Autodesk Inventor part; units mm, degrees
ref_plane "YZ Plane" through (0, 0, 0) normal (1, 0, 0) x (0, 1, 0)
ref_plane "XZ Plane" through (0, 0, 0) normal (0, 1, 0) x (-1, 0, 0)
ref_plane "XY Plane" through (0, 0, 0) normal (0, 0, 1) x (1, 0, 0)
sketch "Sketch1" plane through (0, 0, 0) normal (0, 0, 1) x (1, 0, 0)
  line L0 (0, 0) -> (150, 0)
  line L1 (150, 0) -> (150, -774)
  line L2 (150, -774) -> (0, -774)
  line L3 (0, -774) -> (0, 0)
  dimension "d0" = 150
  dimension "d1" = 774
extrude "Extrusion1" add sketch "Sketch1" along normal blind 4
sketch "Sketch2" plane through (0, 0, 4) normal (0, 0, 1) x (1, 0, 0)
  line L0 (0, 0) -> (0, -774)
  line L1 (0, -150) -> (150, -150)
  line L2 (150, -774) -> (150, 0)
  line L3 (0, -156) -> (150, -156)
  line L4 (150, 0) -> (0, 0)
  line L5 (0, -306) -> (150, -306)
  line L6 (0, -312) -> (150, -312)
  line L7 (0, -462) -> (150, -462)
  line L8 (0, -468) -> (150, -468)
  line L9 (0, -618) -> (150, -618)
  line L10 (0, -624) -> (150, -624)
  line L11 (0, -774) -> (150, -774)
  line L12 (0, -780) -> (150, -780)
  line L13 (75, 0) -> (75, -774)
  line L14 (0, -774) -> (150, -774)
  line L15 (0, 0) -> (0, -774)
  point P0 (75, -306)
  point P1 (75, -618)
  point P2 (75, -156)
  point P3 (75, -150)
  point P4 (75, -312)
  point P5 (75, -306)
  point P6 (75, -468)
  point P7 (75, -462)
  point P8 (75, -624)
  point P9 (75, -618)
  point P10 (75, -780)
  point P11 (75, -774)
  dimension "d4" = 150
  dimension "d5" = 6
  dimension "d6" = 150
  dimension "d8" = 6
  dimension "d9" = 150
  dimension "d10" = 6
  dimension "d11" = 150
  dimension "d12" = 6
  dimension "d13" = 150
  dimension "d14" = 6
extrude "Extrusion2" cut sketch "Sketch2" against normal blind 6 contours L1 L13 L3 L0 | L5 L13 L6 L0 | L7 L13 L8 L0 | L9 L13 L10 L0
properties part number "Separador" material "Wood (Cherry)"
For this review, take the finished solid that the model builds, in its own axes (mm). Give positions to 0.01 mm unless a question says otherwise; leave off trailing zeros. Write each loop counter-clockwise with the first axis right and the second up, starting at its lowest first coordinate (ties: lowest second). Pieces come first, ordered by that corner, then holes. Notation, with made-up numbers: M 13.25,78 L 24.25,78 A9 ccw 24.25,84 Z; hole C 51.5,-25.5 d7. An arc over 180 degrees is marked long. Answer as CSV lines item,"result".
1. Consider section A-A, the plane x = 13. Write out the cut boundary in (y, z).
Findings:
outline,"M -774,0 L -624,0 L -624,4 L -774,4 Z; M -618,0 L -468,0 L -468,4 L -618,4 Z; M -462,0 L -312,0 L -312,4 L -462,4 Z; M -306,0 L -156,0 L -156,4 L -306,4 Z; M -150,0 L 0,0 L 0,4 L -150,4 Z"
2. For pin 1 (1.2 mm diameter, centred on y = -465, z = 3, fed in from -X), flat-tipped, find the tip position at first contact; note if it passes through.
Findings:
pin 1,"stops at x = 75"
3. Wall thickness on line 1 (Y direction, x = 72, z = 0.6): over which ranges is the line inside the solid? List them lowest first.
Findings:
line 1,"y = -774 to -624, -618 to -468, -462 to -312, -306 to -156, -150 to 0"
4. Consider section B-B, the plane z = 3.4. Write out the cut boundary in (x, y), then the cut area to 3 significant figures.
Findings:
outline,"M 0,-774 L 150,-774 L 150,0 L 0,0 L 0,-150 L 75,-150 L 75,-156 L 0,-156 L 0,-306 L 75,-306 L 75,-312 L 0,-312 L 0,-462 L 75,-462 L 75,-468 L 0,-468 L 0,-618 L 75,-618 L 75,-624 L 0,-624 Z"
area,"114,000 mm2"
